```python
from build123d import *

# Parameters (mm, degrees)
SKETCH1_R           = 2
BOSS_EXTRUDE1_DEPTH = 35
SKETCH2_R           = 3.85
BOSS_EXTRUDE2_DEPTH = 3
FILLET1_R           = 1
FILLET2_R           = 1


with BuildPart() as part:
    # Sketch1 → Boss-Extrude1 (new body)
    with BuildSketch(Plane(origin=(0, 0, 0), x_dir=(1, 0, 0), z_dir=(0, 1, 0))):
        Circle(SKETCH1_R)
    extrude(amount=BOSS_EXTRUDE1_DEPTH)

    # Sketch2 → Boss-Extrude2 (add)
    with BuildSketch(Plane(origin=(0, 35, 0), x_dir=(1, 0, 0), z_dir=(0, 1, 0))):
        Circle(SKETCH2_R)
    extrude(amount=BOSS_EXTRUDE2_DEPTH)

    # Fillet1
    fillet1_edges = [part.edges().sort_by_distance(p)[0] for p in [
        (-3.85, 38, 0),
    ]]
    fillet(fillet1_edges, radius=FILLET1_R)

    # Fillet2
    fillet2_edges = [part.edges().sort_by_distance(p)[0] for p in [
        (-2, 0, 0),
        (-2, 35, 0),
    ]]
    fillet(fillet2_edges, radius=FILLET2_R)


solid = part.part
```
Work out the finished part from the listing and answer in its coordinate system (mm). A direction names the side the tool comes from. Round coordinates to 2 decimals unless told otherwise and drop trailing zeros. Write each loop counter-clockwise with the first axis right and the second up, starting at its lowest first coordinate (ties: lowest second). Pieces come first, ordered by that corner, then holes.
1) Flat-ended cylindrical pins translate along their axes: P1, Ø4, axis at y = 19, z = -0.5, coming from the -X side; P2, Ø2.5, axis at x = 0.5, z = -1.5, coming from the -Y side; P3, Ø4, axis at x = 1, y = 5, coming from the -Z side. Find the tip coordinate at first contact, or state that the pin passes through.
2) Which of the six approach directions +Z, -Z, +X, -X, +Y, -Y give full straight-line access (tool end or side, diameter ignored) to faces 1 (the face through (-1, 35, 3)), 2 (the face through (0, 0, 0))?
3) A cutting plane is placed at A-A on y = 16. Determine the outline of the cut face in (x, z), and give its area (3 significant figures).
4) Consider probe 1 along X at (y, z) = (29, 0); probe 2 along Y at (x, z) = (-3, -1). Determine where each line is inside the solid, lowest interval first.
Entries:
1. P1: stops at x = -2
1. P2: stops at y = 0
1. P3: stops at z = -2
2. face 1: -Y
2. face 2: +Z, -Z, +X, -X, -Y
3. outline: circle Ø4 at (0, 0)
3. area: 12.6 mm2
4. probe 1: x = -2 to 2
4. probe 2: y = 35 to 37.95
